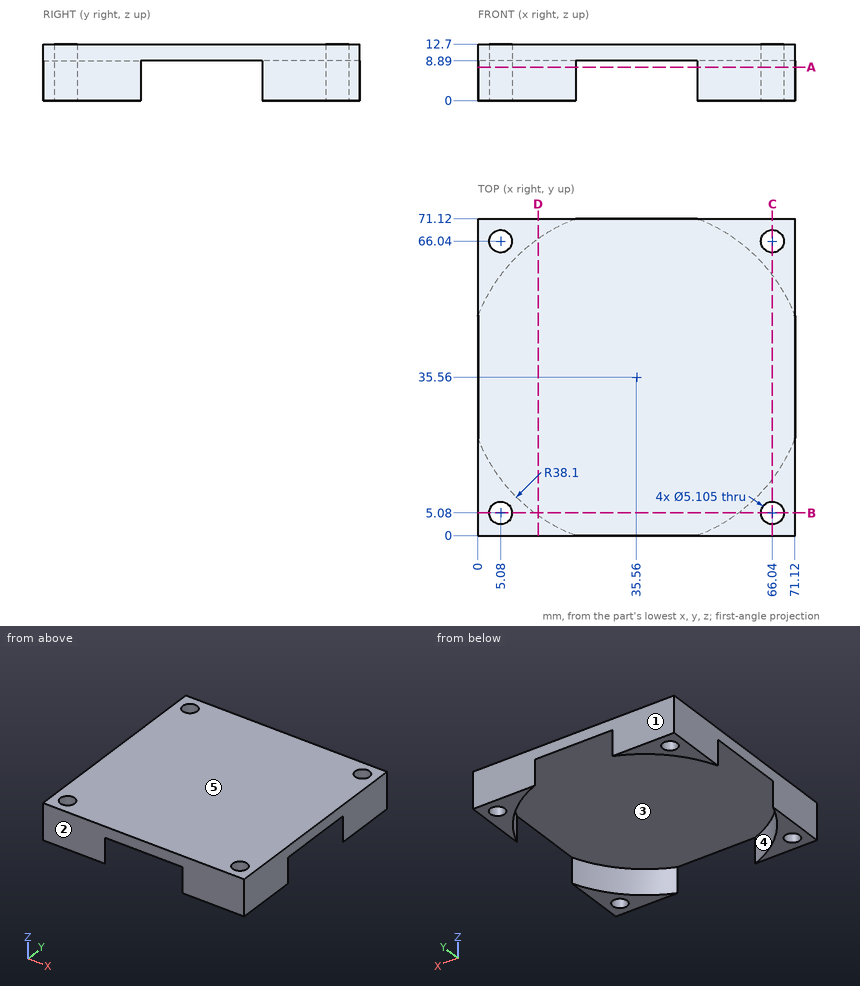
Part print with two shaded views. Sizes in mm from the minimum x, y, z corner. A direction names the side the tool comes from. Round coordinates to 2 decimals unless told otherwise and drop trailing zeros. Order: outer loops, then holes, each group sorted by start corner. A loop starts at its lowest first (then second) coordinate and runs counter-clockwise, first axis right, second up. Notation, with made-up numbers: M -33.75,46.25 L -23.75,46.25 A22 cw -23.75,75.25 Z; hole C -18.75,78.5 d5. An arc over 180 degrees is marked long. Put each result on its own line as item: value. Start each with the question number.
1. Tool access for the marked faces 4 and 5: list every direction of +Z, -Z, +X, -X, +Y, -Y with a clear straight run to the whole face (end or side of a thin tool).
2. Slice it at D-D on x = 13.5. List the corners of the cut face in (y, z), then the cut area to 3 significant figures.
3. Drill centre lines: probe 1 along Y at (x, z) = (5.08, 9.5); probe 2 along Y at (x, z) = (66.04, 6.5) (1 decimal); probe 3 along Z at (x, y) = (57, 15). Where is each one in solid material? Low to high. Write a range as [from, to].
4. Slice it at B-B on y = 5.08. List the corners of the cut face in (x, z), then the cut area to 3 significant figures.
5. Two-plate mould, pull along Y, no slides. Class the marked faces 1, 2 and 3: +Y half, -Y half, draft (parallel to the pull), parting line (faces both ways), or undercut.
6. Drop a flat-ended pin along its axis: pin 1 (2 mm diameter, centred on x = 35.5, y = 11.5, fed in from -Z). Give the stop position or say it passes through.
7. Slice it at A-A on z = 7.5. List the corners of the cut face in (x, y) (1 decimal).
Findings:
1. face 4: -Z
1. face 5: +Z, +X, -X, +Y, -Y
2. outline: M 0,0 L 4.5,0 L 4.5,8.89 L 66.62,8.89 L 66.62,0 L 71.12,0 L 71.12,12.7 L 0,12.7 Z
2. area: 351 mm2
3. probe 1: [0, 2.53], [7.63, 63.49], [68.59, 71.12]
3. probe 2: [0, 2.5], [7.6, 12.7], [58.4, 63.5], [68.6, 71.1]
3. probe 3: [8.89, 12.7]
4. outline: M 0,0 L 2.53,0 L 2.53,12.7 L 0,12.7 Z; M 7.63,0 L 12.7,0 L 12.7,8.89 L 58.42,8.89 L 58.42,0 L 63.49,0 L 63.49,12.7 L 7.63,12.7 Z; M 68.59,0 L 71.12,0 L 71.12,12.7 L 68.59,12.7 Z
4. area: 367 mm2
5. face 1: +Y half
5. face 2: -Y half
5. face 3: undercut
6. pin 1: z = 8.89
7. outline: M 0,0 L 21.9,0 A38.1 cw 0,21.9 Z; M 0,49.2 A38.1 cw 21.9,71.1 L 0,71.1 Z; M 49.2,0 L 71.1,0 L 71.1,21.9 A38.1 cw Z; M 49.2,71.1 A38.1 cw 71.1,49.2 L 71.1,71.1 Z; hole C 5.1,5.1 d5.1; hole C 5.1,66 d5.1; hole C 66,5.1 d5.1; hole C 66,66 d5.1
